Read the model definition and answer for the solid it produces. Units are mm, in the model's axes. Face numbers are marked on the shaded views. A direction names the side the tool comes from. Coordinates: 2 decimals unless noted, no trailing zeros. Write each loop counter-clockwise with the first axis right and the second up, starting at its lowest first coordinate (ties: lowest second). Pieces come first, ordered by that corner, then holes.
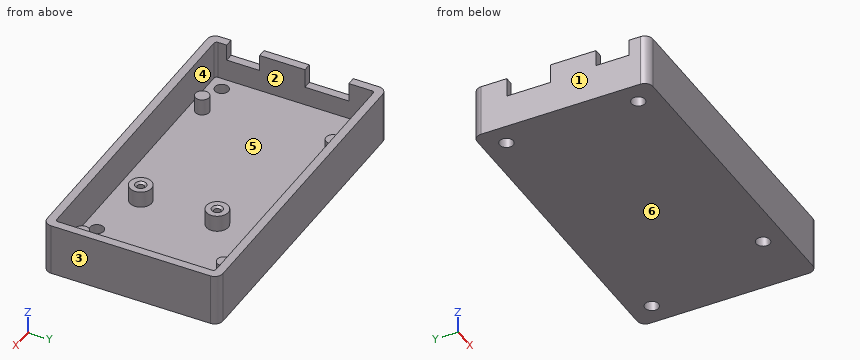
from build123d import *

# Parameters (mm, degrees)
F2_DEPTH       = 5
F4_DEPTH       = 14
F3_R           = 2.5
F3_R_2         = 4
F5_DEPTH       = 6
F7_D           = 2.5
F7_DEPTH       = 6
F7_CSINK_D     = 4
F7_CSINK_ANGLE = 90
F7_TIP         = 0.7510757738
F8_D           = 5
F9_W           = 16
F9_H           = 7
F9_W_2         = 12
F9_H_2         = 6
F10_DEPTH      = 3


# Not quite as in the source:
# - a feature names something its author has since deleted; it is built from what else it names


with BuildPart() as f2:
    # F1 (on Top) → F2 (new body)
    with BuildSketch(Plane.XY):
        with BuildLine():
            ThreePointArc((58, 29), (57.1213203436, 31.1213203436), (55, 32))
            Line((55, 32), (-55, 32))
            ThreePointArc((-55, 32), (-57.1213203436, 31.1213203436), (-58, 29))
            Line((-58, 29), (-58, -29))
            ThreePointArc((-58, -29), (-57.1213203436, -31.1213203436), (-55, -32))
            Line((-55, -32), (55, -32))
            ThreePointArc((55, -32), (57.1213203436, -31.1213203436), (58, -29))
            Line((58, -29), (58, 29))
        make_face()
        with BuildLine():
            ThreePointArc((55, -28), (54.7071067812, -28.7071067812), (54, -29))
            Line((54, -29), (-54, -29))
            ThreePointArc((-54, -29), (-54.7071067812, -28.7071067812), (-55, -28))
            Line((-55, -28), (-55, 28))
            ThreePointArc((-55, 28), (-54.7071067812, 28.7071067812), (-54, 29))
            Line((-54, 29), (54, 29))
            ThreePointArc((54, 29), (54.7071067812, 28.7071067812), (55, 28))
            Line((55, 28), (55, -28))
        make_face(mode=Mode.SUBTRACT)
        with BuildLine():
            Line((-54, -29), (54, -29))
            ThreePointArc((54, -29), (54.7071067812, -28.7071067812), (55, -28))
            Line((55, -28), (55, 28))
            ThreePointArc((55, 28), (54.7071067812, 28.7071067812), (54, 29))
            Line((54, 29), (-54, 29))
            ThreePointArc((-54, 29), (-54.7071067812, 28.7071067812), (-55, 28))
            Line((-55, 28), (-55, -28))
            ThreePointArc((-55, -28), (-54.7071067812, -28.7071067812), (-54, -29))
        make_face()
    extrude(amount=F2_DEPTH)

    # F3 (on face) → F4 (join)
    with BuildSketch(Plane.XY.offset(5)):
        with BuildLine():
            ThreePointArc((58, 29), (57.1213203436, 31.1213203436), (55, 32))
            Line((55, 32), (-55, 32))
            ThreePointArc((-55, 32), (-57.1213203436, 31.1213203436), (-58, 29))
            Line((-58, 29), (-58, -29))
            ThreePointArc((-58, -29), (-57.1213203436, -31.1213203436), (-55, -32))
            Line((-55, -32), (55, -32))
            ThreePointArc((55, -32), (57.1213203436, -31.1213203436), (58, -29))
            Line((58, -29), (58, 29))
        make_face()
        with BuildLine():
            ThreePointArc((55, -28), (54.7071067812, -28.7071067812), (54, -29))
            Line((54, -29), (-54, -29))
            ThreePointArc((-54, -29), (-54.7071067812, -28.7071067812), (-55, -28))
            Line((-55, -28), (-55, 28))
            ThreePointArc((-55, 28), (-54.7071067812, 28.7071067812), (-54, 29))
            Line((-54, 29), (54, 29))
            ThreePointArc((54, 29), (54.7071067812, 28.7071067812), (55, 28))
            Line((55, 28), (55, -28))
        make_face(mode=Mode.SUBTRACT)
    extrude(amount=F4_DEPTH)

    # F3 (on face) → F5 (join)
    with BuildSketch(Plane.XY.offset(5)):
        with BuildLine():
            ThreePointArc((58, 29), (57.1213203436, 31.1213203436), (55, 32))
            Line((55, 32), (-55, 32))
            ThreePointArc((-55, 32), (-57.1213203436, 31.1213203436), (-58, 29))
            Line((-58, 29), (-58, -29))
            ThreePointArc((-58, -29), (-57.1213203436, -31.1213203436), (-55, -32))
            Line((-55, -32), (55, -32))
            ThreePointArc((55, -32), (57.1213203436, -31.1213203436), (58, -29))
            Line((58, -29), (58, 29))
        make_face()
        with BuildLine():
            ThreePointArc((55, -28), (54.7071067812, -28.7071067812), (54, -29))
            Line((54, -29), (-54, -29))
            ThreePointArc((-54, -29), (-54.7071067812, -28.7071067812), (-55, -28))
            Line((-55, -28), (-55, 28))
            ThreePointArc((-55, 28), (-54.7071067812, 28.7071067812), (-54, 29))
            Line((-54, 29), (54, 29))
            ThreePointArc((54, 29), (54.7071067812, 28.7071067812), (55, 28))
            Line((55, 28), (55, -28))
        make_face(mode=Mode.SUBTRACT)
        with Locations((-35.5, 24.15)):
            Circle(F3_R)
        with Locations((-36.8, -24.15)):
            Circle(F3_R)
        with Locations((15.3, 8.95)):
            Circle(F3_R_2)
        with Locations((15.3, -18.95)):
            Circle(F3_R_2)
        with Locations((45.95, -24.15)):
            Circle(F3_R)
        with Locations((39.4, 24.15)):
            Circle(F3_R)
    extrude(amount=F5_DEPTH)

    # F7
    with Locations(Plane.XY.offset(11)):
        with Locations((15.3, 8.95), (15.3, -18.95)):
            CounterSinkHole(F7_D / 2, F7_CSINK_D / 2, depth=F7_DEPTH, counter_sink_angle=F7_CSINK_ANGLE)
            with Locations((0, 0, -(F7_DEPTH + F7_TIP / 2))):  # 118° drill point
                Cone(0, F7_D / 2, F7_TIP, mode=Mode.SUBTRACT)

    # F8 (through all)
    with Locations(Plane.XY.offset(5)):
        with Locations((-50, 24), (50, 24), (35.95, -24), (-50, -24)):
            Hole(F8_D / 2)

    # F9 (on face) → F10 (cut, through all)
    with BuildSketch(Plane(origin=(-58, 0, 0), x_dir=(0, -1, 0), z_dir=(-1, 0, 0))):
        with Locations((-11.65, 15.5)):
            Rectangle(F9_W, F9_H)
        with Locations((18.85, 16)):
            Rectangle(F9_W_2, F9_H_2)
    extrude(amount=-F10_DEPTH, mode=Mode.SUBTRACT)


solid = f2.part
Item 1: For the marked faces 1 and 2, determine the directions among +Z, -Z, +X, -X, +Y, -Y from which every point of the face is accessible in a straight line to the end or side of a thin tool.
Item 2: Find the intervals of material crossed by probe 1 along Y at (x, z) = (15.3, 7.15); probe 2 along Y at (x, z) = (-50, 1.2); probe 3 along X at (y, z) = (-21, 5.75), in increasing order.
Item 3: Determine the mould class of the marked faces 3, 4, 5 and 6 for opening direction X: +X half, -X half, draft (parallel to the pull), parting line (faces both ways), or undercut.
Item 4: The part is cut by section A-A (x = 50). Give the vertices of the cut face in (y, z), and give its area (3 significant figures).
Item 5: Given pin 1 (0.9 mm diameter, centred on x = -56.5, y = 12.5, fed in from +Z); pin 2 (1.5 mm diameter, centred on x = -35.5, y = -23.5, fed in from +Z); pin 3 (6 mm diameter, centred on x = -1.5, y = 6.5, fed in from -Z); pin 4 (6 mm diameter, centred on x = 35.95, y = -24, fed in from +Z), each flat-ended and moving along its own axis, determine where each tip first touches the part or whether it passes through.
Item 6: The part is cut by section B-B (x = -44). Give the vertices of the cut face in (y, z), and give its area (3 significant figures).
Answer:
1. face 1: +Z, -Z, -X, +Y, -Y
1. face 2: +Z
2. probe 1: y = -32 to -29, -22.95 to -20.2, -17.7 to -14.95, 4.95 to 7.7, 10.2 to 12.95, 29 to 32
2. probe 2: y = -32 to -26.5, -21.5 to 21.5, 26.5 to 32
2. probe 3: x = -58 to -55, 11.87 to 18.73, 55 to 58
3. face 3: +X half
3. face 4: undercut
3. face 5: undercut
3. face 6: draft
4. outline: (-32, 0) - (21.5, 0) - (21.5, 5) - (-29, 5) - (-29, 19) - (-32, 19) - close; (26.5, 0) - (32, 0) - (32, 19) - (29, 19) - (29, 5) - (26.5, 5) - close
4. area: 379 mm2
5. pin 1: stops at z = 12
5. pin 2: stops at z = 11
5. pin 3: stops at z = 0
5. pin 4: stops at z = 5
6. outline: (-32, 0) - (32, 0) - (32, 19) - (29, 19) - (29, 5) - (-29, 5) - (-29, 19) - (-32, 19) - close
6. area: 404 mm2
